The listing builds one solid part. Answer for the finished solid, in the listing's coordinates (mm). A direction names the side the tool comes from. Round coordinates to 2 decimals unless told otherwise and drop trailing zeros. Loops run counter-clockwise (first coordinate to the right, second up) from the corner with the lowest first, then second, coordinate; pieces in that order, holes last. Notation, with made-up numbers: (11, -24.5) -> (16, -24.5) arc R14 cw to (16, -14.5) -> close; hole circle Ø9 at (63.25, 10.5). An arc over 180 degrees is marked (long way). Use a Markdown table: item, result. Add a question column.
Q1. For a pull along Z with two mould halves and no side action, classify faces 1 (the flat face through (-42, 27.01, 17)), 2 (the flat face through (-37, 43, 35)), 3 (the cylindrical face through (-22.836, 59.318, 13.064)) as released by +Z, released by -Z, zero draft, split by the parting line, or undercut.
Q2. Consider line 1 (Z direction, x = -32.5, y = 47); line 2 (Y direction, x = -45.5, z = 20); line 3 (X direction, y = 31, z = 19). Determine where each line is inside the solid, lowest interval first.
Q3. Which of the six approach directions +Z, -Z, +X, -X, +Y, -Y give full straight-line access (tool end or side, diameter ignored) to faces 4 (the flat face through (-37, 43, 0)), 5 (the flat face through (-34, 40, 32.5))?
Q4. Section A-A on z = 17.5 is taken. Give the vertices of the cut face in (x, y), then the cut area to 3 significant figures.
Q5. Section D-D on x = -25 is taken. Give the vertices of the cut face in (y, z), then the cut area to 3 significant figures.
Q6. Given pin 1 Ø8 at (y, z) = (48, 19.5) entering from -X; pin 2 Ø8 at (y, z) = (57.01, 17.5) entering from +X; pin 3 Ø15 at (x, z) = (-46, 22) entering from +Y, each flat-ended and moving along its own axis, determine where each tip first touches the part or whether it passes through.
Q7. Section C-C on y = 50.5 is taken. Give the vertices of the cut face in (x, z), then the cut area to 3 significant figures.
Q8. Section B-B on x = -49 is taken. Give the vertices of the cut face in (y, z), then the cut area to 3 significant figures.
from build123d import *

# Parameters (mm, degrees)
F1_DEPTH = 35
F2_T     = -2.5
F3_DEPTH = 25
F4_DEPTH = 25
F6_D     = 10
F8_D     = 10


with BuildPart() as f1:
    # F0 (on Top) → F1 (new body)
    with BuildSketch(Plane.XY):
        with BuildLine():
            Line((-21.6037747636, 67.0103192031), (-29.6037747636, 67.0103192031))
            ThreePointArc((-29.6037747636, 67.0103192031), (-38.9763577657, 44.3829022052), (-61.6037747636, 35.0103192031))
            Line((-61.6037747636, 35.0103192031), (-61.6037747636, 27.0103192031))
            Line((-61.6037747636, 27.0103192031), (-21.6037747636, 27.0103192031))
            Line((-21.6037747636, 27.0103192031), (-21.6037747636, 67.0103192031))
        make_face()
    extrude(amount=F1_DEPTH)

    # F2
    f2_openings = [f1.faces().sort_by_distance(p)[0] for p in [
        (-38.976358, 44.382902, 17.5),
    ]]
    offset(amount=F2_T, openings=f2_openings)

    # F3 (cut): a face of the model
    f3_faces = [f1.faces().sort_by_distance(p)[0] for p in [
        (-26.9026776227, 64.5103192031, 17.5),
    ]]
    extrude(f3_faces, amount=-F3_DEPTH, mode=Mode.SUBTRACT)

    # F4 (cut): a face of the model
    f4_faces = [f1.faces().sort_by_distance(p)[0] for p in [
        (-59.1037747636, 32.3092220622, 17.5),
    ]]
    extrude(f4_faces, amount=-F4_DEPTH, mode=Mode.SUBTRACT)

    # F6 (through all)
    with Locations(Plane(origin=(-24.1037747636, 0, 0), x_dir=(0, -1, 0), z_dir=(-1, 0, 0))):
        with Locations((-57.0103192031, 17.5)):
            Hole(F6_D / 2)

    # F8 (through all)
    with Locations(Plane.XZ.offset(-27.0103192031)):
        with Locations((-51.6037747636, 17.5)):
            Hole(F8_D / 2)


solid = f1.part
Checked values:
| question | item | result |
|---|---|---|
| 1 | face 1 | zero draft |
| 1 | face 2 | released by +Z |
| 1 | face 3 | undercut |
| 2 | line 1 | z = 0 to 2.5, 32.5 to 35 |
| 2 | line 2 | y = 27.01 to 29.51 |
| 2 | line 3 | x = -24.1 to -21.6 |
| 3 | face 4 | -Z, +X, -X, +Y, -Y |
| 3 | face 5 | -X, +Y |
| 4 | outline | (-61.6, 27.01) -> (-56.6, 27.01) -> (-56.6, 29.51) -> (-61.6, 29.51) -> close; (-46.6, 27.01) -> (-21.6, 27.01) -> (-21.6, 52.01) -> (-24.1, 52.01) -> (-24.1, 29.51) -> (-46.6, 29.51) -> close; (-24.1, 62.01) -> (-21.6, 62.01) -> (-21.6, 67.01) -> (-24.1, 67.01) -> close |
| 4 | area | 144 mm2 |
| 5 | outline | (27.01, 0) -> (67.01, 0) -> (67.01, 2.5) -> (29.51, 2.5) -> (29.51, 32.5) -> (67.01, 32.5) -> (67.01, 35) -> (27.01, 35) -> close |
| 5 | area | 275 mm2 |
| 6 | pin 1 | stops at x = -24.1 |
| 6 | pin 2 | passes through |
| 6 | pin 3 | stops at y = 29.51 |
| 7 | outline | (-34.19, 0) -> (-21.6, 0) -> (-21.6, 35) -> (-34.19, 35) -> (-34.19, 32.5) -> (-24.1, 32.5) -> (-24.1, 2.5) -> (-34.19, 2.5) -> close |
| 7 | area | 138 mm2 |
| 8 | outline | (27.01, 0) -> (37.6, 0) -> (37.6, 2.5) -> (29.51, 2.5) -> (29.51, 13.23) -> (27.01, 13.23) -> close; (27.01, 21.77) -> (29.51, 21.77) -> (29.51, 32.5) -> (37.6, 32.5) -> (37.6, 35) -> (27.01, 35) -> close |
| 8 | area | 107 mm2 |
